Work out the finished part from the listing and answer in its coordinate system (mm). Face numbers are marked on the shaded views. Round coordinates to 2 decimals unless told otherwise and drop trailing zeros. Write each loop counter-clockwise with the first axis right and the second up, starting at its lowest first coordinate (ties: lowest second). Pieces come first, ordered by that corner, then holes. Notation, with made-up numbers: M 86,-18 L 96,-18 A21 ccw 96,13 Z; hole C 78,-16.75 d8. An arc over 180 degrees is marked long. Answer in a Markdown table with one row per item.
Solid Edge part; units mm, degrees
sketch "Sketch1" plane through (0, 0, 0) normal (0, 0, 1) x (1, 0, 0)
  line L0 (52.05, -45.35) -> (-52.05, -45.35)
  line L1 (-52.05, -45.35) -> (-52.05, 45.35)
  line L2 (-52.05, 45.35) -> (52.05, 45.35)
  line L3 (52.05, 45.35) -> (52.05, -45.35)
extrude "Protrusion1" add sketch "Sketch1" against normal blind 5
sketch "Sketch2" plane through (0, 0, 0) normal (0, 0, 1) x (1, 0, 0)
  line L0 (-47.05, -40.35) -> (-47.05, 40.35)
  line L1 (-47.05, 40.35) -> (47.05, 40.35)
  line L2 (47.05, 40.35) -> (47.05, -40.35)
  line L3 (47.05, -40.35) -> (-47.05, -40.35)
extrude "ExtrudedCutout_1" cut sketch "Sketch2" against normal blind 1.5
sketch "Sketch3" plane through (0, 0, -1.5) normal (0, 0, 1) x (1, 0, 0)
  line L0 (-6.26, -13.93) -> (-16.26, -13.93)
  line L1 (-16.26, -13.93) -> (-23.26, -6.93)
  line L2 (-23.26, -6.93) -> (-23.26, 9.07)
  line L3 (-23.26, 9.07) -> (-21.76, 10.57)
  line L4 (-21.76, 10.57) -> (-9.26, 10.57)
  line L5 (-9.26, 10.57) -> (-7.76, 9.07)
  line L6 (-7.76, 9.07) -> (6.74, 9.07)
  line L7 (6.74, 9.07) -> (8.24, 10.57)
  line L8 (8.24, 10.57) -> (13.74, 10.57)
  line L9 (13.74, 10.57) -> (17.74, 6.57)
  line L10 (17.74, 6.57) -> (17.74, -4.43)
  line L11 (17.74, -4.43) -> (11.24, -10.93)
  line L12 (11.24, -10.93) -> (-3.26, -10.93)
  line L13 (-3.26, -10.93) -> (-6.26, -13.93)
extrude "ExtrudedCutout_2" cut sketch "Sketch3" against normal blind 2
sketch "Sketch4" plane through (0, 0, -1.5) normal (0, 0, 1) x (1, 0, 0)
  line L0 (-20.76, -1.43) -> (-25.76, -1.43)
  line L1 (-25.76, -1.43) -> (-25.76, 3.57)
  line L2 (-25.76, 3.57) -> (-20.76, 3.57)
  line L3 (-20.76, 3.57) -> (-20.76, -1.43)
  line L4 (-19.76, -13.9655) -> (-16.2245, -10.43)
  line L5 (-16.2245, -10.43) -> (-19.76, -6.8945)
  line L6 (-19.76, -6.8945) -> (-23.2955, -10.43)
  line L7 (-23.2955, -10.43) -> (-19.76, -13.9655)
  line L8 (-15.0977, -11.43) -> (-10.0977, -11.43)
  line L9 (-10.0977, -11.43) -> (-10.0977, -16.43)
  line L10 (-10.0977, -16.43) -> (-15.0977, -16.43)
  line L11 (-15.0977, -16.43) -> (-15.0977, -11.43)
  line L12 (-13.01, 8.07) -> (-13.01, 13.07)
  line L13 (-13.01, 13.07) -> (-18.01, 13.07)
  line L14 (-18.01, 13.07) -> (-18.01, 8.07)
  line L15 (-18.01, 8.07) -> (-13.01, 8.07)
  line L16 (9.6793, -8.0539) -> (9.6793, -13.8061)
  line L17 (9.6793, -13.8061) -> (3.927, -13.8061)
  line L18 (3.927, -13.8061) -> (3.927, -8.0539)
  line L19 (3.927, -8.0539) -> (9.6793, -8.0539)
  line L20 (14.49, -11.2155) -> (18.0255, -7.68)
  line L21 (18.0255, -7.68) -> (14.49, -4.1445)
  line L22 (14.49, -4.1445) -> (10.9545, -7.68)
  line L23 (10.9545, -7.68) -> (14.49, -11.2155)
  line L24 (20.24, 2.6121) -> (20.24, 7.6121)
  line L25 (20.24, 7.6121) -> (15.24, 7.6121)
  line L26 (15.24, 7.6121) -> (15.24, 2.6121)
  line L27 (15.24, 2.6121) -> (20.24, 2.6121)
  line L28 (1.99, 11.57) -> (-3.01, 11.57)
  line L29 (-3.01, 11.57) -> (-3.01, 6.57)
  line L30 (-3.01, 6.57) -> (1.99, 6.57)
  line L31 (1.99, 6.57) -> (1.99, 11.57)
extrude "Cutout1" cut sketch "Sketch4" against normal through all
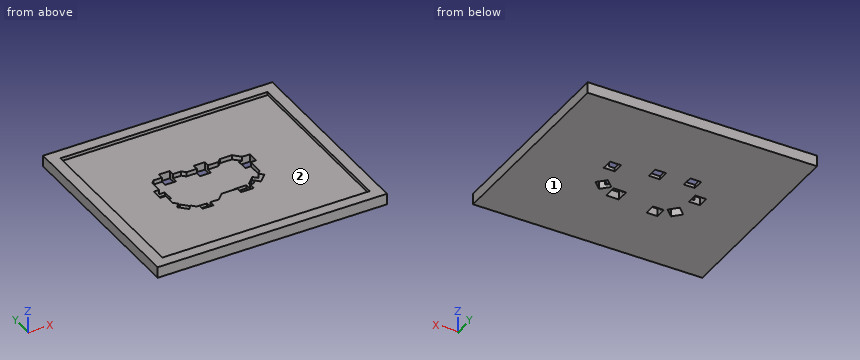
1. Consider line 1 along Y through (x, z) = (-12, -3.1); line 2 along X through (y, z) = (9, -4.3); line 3 along Y through (x, z) = (23.5, -0.25). Determine where each line is inside the solid, lowest interval first. Write a range as from..to.
Calculated:
| item | result |
|---|---|
| line 1 | y = -45.35..-16.43, 10.57..45.35 |
| line 2 | x = -52.05..-18.01, -13.01..-3.01, 1.99..52.05 |
| line 3 | y = -45.35..-40.35, 40.35..45.35 |
2. The part is cut by section A-A (y = -32). Determine the outline of the cut face in (x, z), plus the area to 3 significant figures.
Calculated:
| item | result |
|---|---|
| outline | M -52.05,-5 L 52.05,-5 L 52.05,0 L 47.05,0 L 47.05,-1.5 L -47.05,-1.5 L -47.05,0 L -52.05,0 Z |
| area | 379 mm² |
3. The part is cut by section C-C (z = -4.25). Count the separate pieces of the cut face and the enclosed holes in it, plus the area to 3 significant figures.
Calculated:
| item | result |
|---|---|
| separate pieces | 1 |
| enclosed holes | 8 |
| area | 9,230 mm² |
4. The part is cut by section B-B (x = 22). Determine the outline of the cut face in (y, z), plus the area to 3 significant figures.
Calculated:
| item | result |
|---|---|
| outline | M -45.35,-5 L 45.35,-5 L 45.35,0 L 40.35,0 L 40.35,-1.5 L -40.35,-1.5 L -40.35,0 L -45.35,0 Z |
| area | 332 mm² |
5. Given pin 1 (12 mm diameter, centred on x = 1, y = -3.5, fed in from +Z); pin 2 (12 mm diameter, centred on x = -7, y = -27, fed in from +Z), each flat-ended and moving along its own axis, determine where each tip first touches the part or whether it passes through.
Calculated:
| item | result |
|---|---|
| pin 1 | stops at z = -3.5 |
| pin 2 | stops at z = -1.5 |
6. Determine the mould class of the marked faces 1 and 2 for opening direction X: released by +X, released by -X, zero draft, split by the parting line, or undercut.
Calculated:
| item | result |
|---|---|
| face 1 | zero draft |
| face 2 | undercut |
